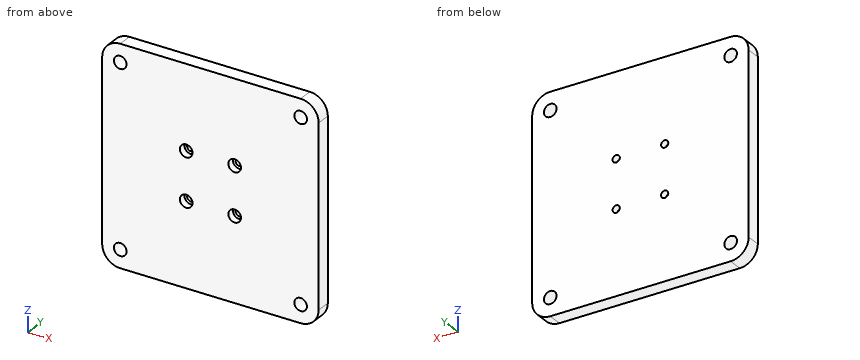
from build123d import *

# Parameters (mm, degrees)
SKETCH_1_W          = 120
SKETCH_1_H          = 120
SKETCH_1_R          = 2
EXTRUDE_1_DEPTH     = 8
SKETCH_2_R          = 3.5
CUT_EXTRUDE_1_DEPTH = 10
SKETCH_3_R          = 3.5
CUT_EXTRUDE_2_DEPTH = 4
FILLET_1_R          = 10


with BuildPart() as part:
    # 草图1 → 凸台-拉伸1 (new body)
    with BuildSketch(Plane(origin=(0, 0, 0), x_dir=(1, 0, 0), z_dir=(0, 1, 0))):
        Rectangle(SKETCH_1_W, SKETCH_1_H)
        with Locations((-13.435028843, 13.435028843)):
            Circle(SKETCH_1_R, mode=Mode.SUBTRACT)
        with Locations((13.435028843, 13.435028843)):
            Circle(SKETCH_1_R, mode=Mode.SUBTRACT)
        with Locations((13.435028843, -13.435028843)):
            Circle(SKETCH_1_R, mode=Mode.SUBTRACT)
        with Locations((-13.435028843, -13.435028843)):
            Circle(SKETCH_1_R, mode=Mode.SUBTRACT)
    extrude(amount=EXTRUDE_1_DEPTH)

    # 草图2 → 切除-拉伸1 (cut)
    with BuildSketch(Plane(origin=(0, 8, 0), x_dir=(1, 0, 0), z_dir=(0, 1, 0))):
        with Locations((-50, 50)):
            Circle(SKETCH_2_R)
        with Locations((50, 50)):
            Circle(SKETCH_2_R)
        with Locations((50, -50)):
            Circle(SKETCH_2_R)
        with Locations((-50, -50)):
            Circle(SKETCH_2_R)
    extrude(amount=-CUT_EXTRUDE_1_DEPTH, mode=Mode.SUBTRACT)

    # 草图3 → 切除-拉伸2 (cut)
    with BuildSketch(Plane.XZ):
        with Locations((-13.435028843, 13.435028843)):
            Circle(SKETCH_3_R)
        with Locations((13.435028843, 13.435028843)):
            Circle(SKETCH_3_R)
        with Locations((-13.435028843, -13.435028843)):
            Circle(SKETCH_3_R)
        with Locations((13.435028843, -13.435028843)):
            Circle(SKETCH_3_R)
    extrude(amount=-CUT_EXTRUDE_2_DEPTH, mode=Mode.SUBTRACT)

    # 圆角1
    fillet_1_edges = [part.edges().sort_by_distance(p)[0] for p in [
        (60, 4, 60),
        (-60, 4, 60),
        (-60, 4, -60),
        (60, 4, -60),
    ]]
    fillet(fillet_1_edges, radius=FILLET_1_R)


solid = part.part
Work out the finished part from the listing and answer in its coordinate system (mm). Round coordinates to 2 decimals unless told otherwise and drop trailing zeros. Write each question's results on one line, items separated by ' | '.
Item 1: Find the intervals of material crossed by line 1 along X through (y, z) = (3.5, -50); line 2 along Z through (x, y) = (52.5, 6); line 3 along X through (y, z) = (7.25, 14.5), in increasing order. Write a range as [from, to].
Result set:
line 1: [-60, -53.5], [-46.5, 46.5], [53.5, 60] | line 2: [-59.68, -52.45], [-47.55, 47.55], [52.45, 59.68] | line 3: [-60, -15.13], [-11.74, 11.74], [15.13, 60]
Item 2: A flat-ended cylindrical pin translates along its axis: P1, Ø6.5, axis at x = 13.44, z = 13.44, coming from the -Y side. Find the tip coordinate at first contact, or state that the pin passes through.
Result set:
P1: y = 4
Item 3: A cutting plane is placed at A-A, the plane y = 6. Count the separate pieces of the cut face and the enclosed holes in it, plus the area to 3 significant figures.
Result set:
separate pieces: 1 | enclosed holes: 8 | area: 14,100 mm^2
